```python
from build123d import *

# Parameters (mm, degrees)
SKETCH_1_W      = 68
SKETCH_1_H      = 50
SKETCH_1_R      = 12
SKETCH_1_R_2    = 1.6
EXTRUDE_1_DEPTH = 5


with BuildPart() as part:
    # 草图1 → 凸台-拉伸1 (new body)
    with BuildSketch(Plane(origin=(0, 0, 0), x_dir=(1, 0, 0), z_dir=(0, 1, 0))):
        with Locations((34, -25)):
            Rectangle(SKETCH_1_W, SKETCH_1_H)
        with Locations(Location((41, -25, 0), (0, 0, 270))):
            Circle(SKETCH_1_R, mode=Mode.SUBTRACT)
        with Locations(Location((25.5, -9.5, 0), (0, 0, 270))):
            Circle(SKETCH_1_R_2, mode=Mode.SUBTRACT)
        with Locations(Location((56.5, -9.5, 0), (0, 0, 270))):
            Circle(SKETCH_1_R_2, mode=Mode.SUBTRACT)
        with Locations(Location((56.5, -40.5, 0), (0, 0, 270))):
            Circle(SKETCH_1_R_2, mode=Mode.SUBTRACT)
        with Locations(Location((25.5, -40.5, 0), (0, 0, 270))):
            Circle(SKETCH_1_R_2, mode=Mode.SUBTRACT)
        with BuildLine():
            Line((8, -6.5), (10, -6.5))
            ThreePointArc((10, -6.5), (12.5, -9), (10, -11.5))
            Line((10, -11.5), (8, -11.5))
            ThreePointArc((8, -11.5), (5.5, -9), (8, -6.5))
        make_face(mode=Mode.SUBTRACT)
        with BuildLine():
            Line((8, -38.5), (10, -38.5))
            ThreePointArc((10, -38.5), (12.5, -41), (10, -43.5))
            Line((10, -43.5), (8, -43.5))
            ThreePointArc((8, -43.5), (5.5, -41), (8, -38.5))
        make_face(mode=Mode.SUBTRACT)
    extrude(amount=EXTRUDE_1_DEPTH)


solid = part.part
```
Design review of the part built by this model. Coordinates are the model's own, in mm. A direction names the side the tool comes from. Coordinates: 2 decimals unless noted, no trailing zeros. Write each loop counter-clockwise with the first axis right and the second up, starting at its lowest first coordinate (ties: lowest second). Pieces come first, ordered by that corner, then holes.
1) Mouldability with a two-part tool opening along X and no side actions: class faces 1 (the flat face through (34, 2, 50)), 2 (the flat face through (0, 2, 25)), 3 (the cylindrical face through (12.5, 2.5, 40.9)) as +X half, -X half, draft (parallel to the pull), parting line (faces both ways), or undercut.
2) Add section A-A (x = 56.5). Write out the cut boundary in (y, z), plus the area to 3 significant figures.
3) Add section C-C (y = 0.75). Write out the cut boundary in (x, z), plus the area to 3 significant figures.
4) Insertion check: pin 1 (1 mm diameter, centred on x = 18, y = 2, fed in from -Z). The pin has a flat end and moves straight along its axis. Give the tip position at first contact, or say it passes through.
5) Add section B-B (z = 25). Write out the cut boundary in (x, y), plus the area to 3 significant figures.
6) Add section D-D (z = 9). Write out the cut boundary in (x, y).
7) Machinability: for faces 4 (the flat face through (9, 2, 43.5)), 5 (the flat face through (26, 0, 25)), which of the approach directions +Z, -Z, +X, -X, +Y, -Y give a long, thin tool a straight path to every point of the face, cutting with its end or side? Answer none if there is none.
8) To check wall thickness, follow L1, parallel to X at y = 1.1, z = 40; L2, parallel to Z at x = 25, y = 2.8; L3, parallel to X at y = 3.8, z = 25. State the ranges of each line that lie inside material, in increasing order.
Check result:
1. face 1: draft
1. face 2: -X half
1. face 3: undercut
2. outline: (0, 0) - (5, 0) - (5, 7.9) - (0, 7.9) - close; (0, 11.1) - (5, 11.1) - (5, 38.9) - (0, 38.9) - close; (0, 42.1) - (5, 42.1) - (5, 50) - (0, 50) - close
2. area: 218 mm2
3. outline: (0, 0) - (68, 0) - (68, 50) - (0, 50) - close; hole (8, 6.5) - (10, 6.5) arc R2.5 ccw to (10, 11.5) - (8, 11.5) arc R2.5 ccw to start; hole (8, 38.5) - (10, 38.5) arc R2.5 ccw to (10, 43.5) - (8, 43.5) arc R2.5 ccw to start; hole circle Ø3.2 at (25.5, 9.5); hole circle Ø3.2 at (25.5, 40.5); hole circle Ø24 at (41, 25); hole circle Ø3.2 at (56.5, 9.5); hole circle Ø3.2 at (56.5, 40.5)
3. area: 2,860 mm2
4. pin 1: stops at z = 0
5. outline: (0, 0) - (29, 0) - (29, 5) - (0, 5) - close; (53, 0) - (68, 0) - (68, 5) - (53, 5) - close
5. area: 220 mm2
6. outline: (0, 0) - (5.5, 0) - (5.5, 5) - (0, 5) - close; (12.5, 0) - (23.98, 0) - (23.98, 5) - (12.5, 5) - close; (27.02, 0) - (54.98, 0) - (54.98, 5) - (27.02, 5) - close; (58.02, 0) - (68, 0) - (68, 5) - (58.02, 5) - close
7. face 4: +Y, -Y
7. face 5: +Z, -Z, +X, -X, -Y
8. L1: x = 0 to 5.71, 12.29 to 23.98, 27.02 to 54.98, 58.02 to 68
8. L2: z = 0 to 7.98, 11.02 to 38.98, 42.02 to 50
8. L3: x = 0 to 29, 53 to 68
